For this review, take the finished solid that the model builds, in its own axes (mm). Give positions to 0.01 mm unless a question says otherwise; leave off trailing zeros. Order: outer loops, then holes, each group sorted by start corner. A loop starts at its lowest first (then second) coordinate and runs counter-clockwise, first axis right, second up. Notation, with made-up numbers: M -29.75,83.5 L 15.25,83.5 A36 ccw 15.25,118.5 Z; hole C -6.5,47.5 d6. An arc over 180 degrees is marked long. Use CSV: the item, a comma, the result in double quotes. Start each with the question number.
(1) Consider section B-B (y = -413.5). Write out the cut boundary in (x, z).
(2) Clearance check with flat-ended pins moving along their axes: P1, Ø0.8, axis at y = -570.5, z = 55.5, coming from the +X side; P2, Ø9, axis at x = -63.45, y = -748.81, coming from the -Z side; P3, Ø0.8, axis at y = -318, z = 56, coming from the -X side. State where each tip first meets the part, or that it passes through.
(3) Wall thickness on L1, parallel to X at y = -319, z = 46; L2, parallel to Z at x = -47.5, y = -527; L3, parallel to Z at x = -64, y = -367: over which ranges is each line inside the solid? List them lowest first. Write a range as from..to.
(4) Consider section A-A (z = 49.5). Write out the cut boundary in (x, y).
```python
from build123d import *

# Parameters (mm, degrees)
F1_DEPTH = 768.81
F3_D     = 11


with BuildPart() as f1:
    # F0 (on Front) → F1 (new body)
    with BuildSketch(Plane.XZ):
        with BuildLine():
            ThreePointArc((-83.451096, 34.500868), (-82.86531, 33.086655), (-81.451096, 32.500868))
            Line((-81.451096, 32.500868), (-45.451096, 32.500868))
            ThreePointArc((-45.451096, 32.500868), (-44.036883, 33.086655), (-43.451096, 34.500868))
            Line((-43.451096, 34.500868), (-43.451096, 54.500868))
            ThreePointArc((-43.451096, 54.500868), (-44.036883, 55.915082), (-45.451096, 56.500868))
            Line((-45.451096, 56.500868), (-53.451096, 56.500868))
            Line((-53.451096, 56.500868), (-53.451096, 55.000868))
            Line((-53.451096, 55.000868), (-45.951096, 55.000868))
            ThreePointArc((-45.951096, 55.000868), (-45.24399, 54.707975), (-44.951096, 54.000868))
            Line((-44.951096, 54.000868), (-44.951096, 35.000868))
            ThreePointArc((-44.951096, 35.000868), (-45.24399, 34.293762), (-45.951096, 34.000868))
            Line((-45.951096, 34.000868), (-80.951096, 34.000868))
            ThreePointArc((-80.951096, 34.000868), (-81.658203, 34.293762), (-81.951096, 35.000868))
            Line((-81.951096, 35.000868), (-81.951096, 54.000868))
            ThreePointArc((-81.951096, 54.000868), (-81.658203, 54.707975), (-80.951096, 55.000868))
            Line((-80.951096, 55.000868), (-73.451096, 55.000868))
            Line((-73.451096, 55.000868), (-73.451096, 56.500868))
            Line((-73.451096, 56.500868), (-81.451096, 56.500868))
            ThreePointArc((-81.451096, 56.500868), (-82.86531, 55.915082), (-83.451096, 54.500868))
            Line((-83.451096, 54.500868), (-83.451096, 34.500868))
        make_face()
    extrude(amount=F1_DEPTH)

    # F3 (through all)
    with Locations(Plane(origin=(0, 0, 32.500868), x_dir=(1, 0, 0), z_dir=(0, 0, -1))):
        with Locations((-63.451096, 748.81), (-63.451096, 20)):
            Hole(F3_D / 2)


solid = f1.part
```
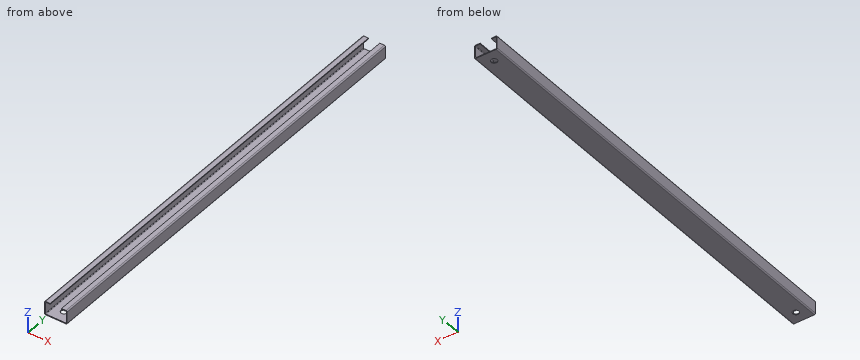
Check result:
1,outline,"M -83.45,34.5 A2 ccw -81.45,32.5 L -45.45,32.5 A2 ccw -43.45,34.5 L -43.45,54.5 A2 ccw -45.45,56.5 L -53.45,56.5 L -53.45,55 L -45.95,55 A1 cw -44.95,54 L -44.95,35 A1 cw -45.95,34 L -80.95,34 A1 cw -81.95,35 L -81.95,54 A1 cw -80.95,55 L -73.45,55 L -73.45,56.5 L -81.45,56.5 A2 ccw -83.45,54.5 Z"
2,P1,"stops at x = -43.54"
2,P2,"passes through"
2,P3,"stops at x = -83.12"
3,L1,"x = -83.45..-81.95, -44.95..-43.45"
3,L2,"z = 32.5..34, 55..56.5"
3,L3,"z = 32.5..34"
4,outline,"M -83.45,-768.81 L -81.95,-768.81 L -81.95,0 L -83.45,0 Z; M -44.95,-768.81 L -43.45,-768.81 L -43.45,0 L -44.95,0 Z"
